Source: CAD feature listing. Evaluate the final solid. Frame: model axes, mm. Face numbers are marked on the shaded views. A direction names the side the tool comes from. Give positions to 0.01 mm unless a question says otherwise; leave off trailing zeros. Order: outer loops, then holes, each group sorted by start corner. A loop starts at its lowest first (then second) coordinate and runs counter-clockwise, first axis right, second up. Notation, with made-up numbers: (85, -15.75) - (97, -15.75) arc R28 cw to (97, 14.25) - close; hole circle Ø10 at (41.25, 1.25). An arc over 180 degrees is marked (long way). One line per item, written item: value. Start each with the question number.
from build123d import *

# Parameters (mm, degrees)
EXTRUDE_1_DEPTH     = 23
SKETCH_5_R          = 2.7
SKETCH_5_R_2        = 4.75
EXTRUDE_6_DEPTH     = 7
SKETCH_6_R          = 2.15
CUT_EXTRUDE_2_DEPTH = 78.35709986
SKETCH_8_W          = 20.5
SKETCH_8_H          = 16.823085553
CUT_EXTRUDE_4_DEPTH = 7
SKETCH_14_W         = 13.6
SKETCH_14_H         = 4.3
CUT_EXTRUDE_7_DEPTH = 22.74


with BuildPart() as part:
    # Эскиз1 → Бобышка-Вытянуть1 (new body)
    with BuildSketch(Plane.XY):
        Polygon((-59.190561798, -40.176897727), (-59.190561798, -15.085730337), (-51.190561798, -15.085730337), (-51.190561798, -38.085730337), (-10.190561798, -38.085730337), (-10.190561798, -15.085730337), (-2.190561798, -15.085730337), (-2.190561798, -38.085730337), (-2.190561798, -44.176897727), (-59.190561798, -44.176897727), align=None)
    extrude(amount=EXTRUDE_1_DEPTH)

    # Эскиз5 → Бобышка-Вытянуть6 (add)
    with BuildSketch(Plane.XY.offset(23)):
        Polygon((-21.190561798, -19.58573034), (-51.190561798, -19.58573034), (-51.190561798, -34.983929743), (-51.190561798, -38.085730337), (-10.190561798, -38.085730337), (-10.190561798, -34.983929743), (-10.190561798, -19.58573034), align=None)
        with Locations((-21.190561798, -28.085730337)):
            Circle(SKETCH_5_R, mode=Mode.SUBTRACT)
        with Locations(Location((-40.190561798, -28.085730337, 0), (0, 0, 180))):
            Circle(SKETCH_5_R_2, mode=Mode.SUBTRACT)
    extrude(amount=-EXTRUDE_6_DEPTH)

    # Эскиз6 → Вырез-Вытянуть2 (cut, through all)
    with BuildSketch(Plane.XY.offset(23)):
        with Locations((-6.040561798, -33.885730337)):
            Circle(SKETCH_6_R)
        with Locations((-6.040561798, -22.285730337)):
            Circle(SKETCH_6_R)
        with Locations((-55.340561798, -33.885730337)):
            Circle(SKETCH_6_R)
        with Locations((-55.340561798, -22.285730337)):
            Circle(SKETCH_6_R)
    extrude(amount=-CUT_EXTRUDE_2_DEPTH, mode=Mode.SUBTRACT)

    # Эскиз8 → Вырез-Вытянуть4 (cut)
    with BuildSketch(Plane.XY.offset(23)):
        with Locations((-20.440561798, -27.997273117)):
            Rectangle(SKETCH_8_W, SKETCH_8_H)
    extrude(amount=-CUT_EXTRUDE_4_DEPTH, mode=Mode.SUBTRACT)

    # Эскиз14 → Вырез-Вытянуть7 (cut)
    with BuildSketch(Plane(origin=(0, -44.176897727, 0), x_dir=(-1, 0, 0), z_dir=(0, -1, 0))):
        with Locations((40.227814592, -19.162885498)):
            Rectangle(SKETCH_14_W, SKETCH_14_H)
    extrude(amount=-CUT_EXTRUDE_7_DEPTH, mode=Mode.SUBTRACT)


solid = part.part
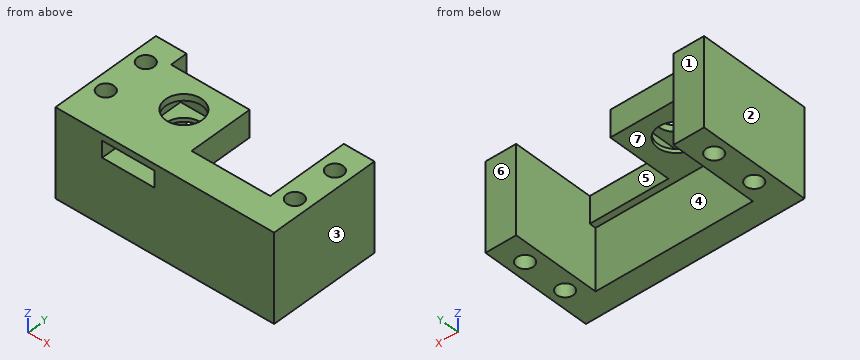
1. Section B-B on x = -43.5. Return the cut outline in (y, z), then the cut area to 3 significant figures.
2. Section A-A on z = 3.75. Return the cut outline in (x, y).
3. Contact query for flat-ended pins moving along their axis: pin 1 Ø4 at (x, y) = (-55.34, -33.89) entering from +Z; pin 2 Ø10 at (x, y) = (-28, -19) entering from -Z; pin 3 Ø5.5 at (x, z) = (-16.5, 18.5) entering from +Y; pin 4 Ø7 at (x, y) = (-39, -35.5) entering from -Z. Output: stop coordinate, or through.
4. Section D-D on x = -16. Return the cut outline in (y, z).
5. Ray query, L1, parallel to Y at x = -6, z = 8; L2, parallel to Y at x = -8, z = 21.75; L3, parallel to Z at x = -45, y = -42. Return the intervals inside material, ascending.
6. Set-up query: the marked faces 5, 6 and 7. Return all of +Z, -Z, +X, -X, +Y, -Y with unobstructed straight access to the full face (end or side cutting, diameter ignored); none if empty.
7. Draft query along X for the marked faces 1, 2, 3 and 4. Return one class per face: pulls with the +X half, pulls with the -X half, needs draft (parallel to the pull), parting line crosses it, or undercut.
8. Section C-C on y = -26.5. Return the cut outline in (x, z), then the cut area to 3 significant figures.
Data:
1. outline: (-44.18, 0) - (-38.09, 0) - (-38.09, 16) - (-31.49, 16) - (-31.49, 17.01) - (-44.18, 17.01) - close; (-44.18, 21.31) - (-31.49, 21.31) - (-31.49, 23) - (-44.18, 23) - close; (-24.68, 16) - (-19.59, 16) - (-19.59, 23) - (-24.68, 23) - (-24.68, 21.31) - (-21.44, 21.31) - (-21.44, 17.01) - (-24.68, 17.01) - close
1. area: 153 mm2
2. outline: (-59.19, -44.18) - (-2.19, -44.18) - (-2.19, -15.09) - (-10.19, -15.09) - (-10.19, -38.09) - (-51.19, -38.09) - (-51.19, -15.09) - (-59.19, -15.09) - close; hole circle Ø4.3 at (-55.34, -33.89); hole circle Ø4.3 at (-55.34, -22.29); hole circle Ø4.3 at (-6.04, -33.89); hole circle Ø4.3 at (-6.04, -22.29)
3. pin 1: passes through
3. pin 2: stops at z = 16
3. pin 3: stops at y = -36.41
3. pin 4: stops at z = 0
4. outline: (-44.18, 0) - (-38.09, 0) - (-38.09, 16) - (-36.41, 16) - (-36.41, 23) - (-44.18, 23) - close
5. L1: y = -44.18 to -36.04, -31.74 to -24.44, -20.14 to -15.09
5. L2: y = -44.18 to -34.77, -33 to -23.17, -21.4 to -15.09
5. L3: z = 0 to 17.01, 21.31 to 23
6. face 5: +Z, -Z, +Y
6. face 6: +Z, -Z, +X, -X, +Y
6. face 7: -Z, +Y
7. face 1: needs draft
7. face 2: pulls with the -X half
7. face 3: pulls with the +X half
7. face 4: undercut
8. outline: (-59.19, 0) - (-51.19, 0) - (-51.19, 16) - (-44.67, 16) - (-44.67, 17.01) - (-47.03, 17.01) - (-47.03, 21.31) - (-44.67, 21.31) - (-44.67, 23) - (-59.19, 23) - close; (-35.71, 16) - (-30.69, 16) - (-30.69, 23) - (-35.71, 23) - (-35.71, 21.31) - (-33.43, 21.31) - (-33.43, 17.01) - (-35.71, 17.01) - close; (-10.19, 0) - (-2.19, 0) - (-2.19, 23) - (-10.19, 23) - close
8. area: 429 mm2
